Geometry check sheet. Reference: the model listing, model coordinates, mm. A direction names the side the tool comes from. Give positions to 0.01 mm unless a question says otherwise; leave off trailing zeros. Loops run counter-clockwise (first coordinate to the right, second up) from the corner with the lowest first, then second, coordinate; pieces in that order, holes last. Notation, with made-up numbers: (81.25, 9) - (140.25, 9) arc R18 ccw to (140.25, 13) - close; hole circle Ø11 at (73.5, 6.5). An arc over 180 degrees is marked (long way). Use a Markdown table: item, result. Add a question column.
1. Cross-section at D-D on x = 6.5. Enter the section's corners in (y, z).
2. Cross-section at A-A on x = 0. Enter the section's corners in (y, z), and give its area (3 significant figures).
3. Depth check by flat-ended pin: P1, Ø3, axis at y = 11.5, z = 14.5, coming from the +X side; P2, Ø5, axis at y = 6.5, z = 12.5, coming from the +X side; P3, Ø4, axis at x = -4.5, z = 3.5, coming from the +Y side. Enter the tip coordinate at first touch or a pass-through.
4. Cross-section at B-B on z = 6.75. Enter the section's corners in (x, y), and give its area (3 significant figures).
5. Draft check along Z on faces 5 (the flat face through (12, -9, 15.4)), 6 (the flat face through (-4, -4, 0)), 7 (the flat face through (13.16, -6.78, 19.34)). Enter one of: pulls with the +Z half, pulls with the -Z half, needs draft (parallel to the pull), parting line crosses it, or undercut.
6. Cross-section at C-C on y = -0.5. Enter the section's corners in (x, z).
7. Material ranges on L1, parallel to X at y = -0.5, z = 9.5; L2, parallel to Y at x = 0, z = 3.5; L3, parallel to Y at x = 0, z = 9.5, recorded low to high.
8. Set-up check for faces 1 (the flat face through (-15, 2.25, 19)), 2 (the cylindrical face through (13.94, -10.16, 19.34)), 3 (the flat face through (-15, -2.25, 19)), 4 (the flat face through (-12, -4, 5)): record each of +Z, -Z, +X, -X, +Y, -Y from which the full face is reachable in a straight line by a thin tool's end or side.
from build123d import *

# Parameters (mm, degrees)
F0_R     = 17.5
F0_R_2   = 5.5
F1_DEPTH = 5
F2_R     = 12.3
F2_R_2   = 5.5
F3_DEPTH = 10.4
F5_DEPTH = 8


with BuildPart() as f1:
    # F0 (on Top) → F1 (new body)
    with BuildSketch(Plane.XY):
        Circle(F0_R)
        Circle(F0_R_2, mode=Mode.SUBTRACT)
    extrude(amount=F1_DEPTH)

    # F2 (on face) → F3 (join)
    with BuildSketch(Plane.XY.offset(5)):
        Circle(F2_R)
        Circle(F2_R_2, mode=Mode.SUBTRACT)
    extrude(amount=F3_DEPTH)

    # F4 (on face) → F5 (join)
    with BuildSketch(Plane.XY.offset(15.4)):
        with BuildLine():
            Line((-1.5968973469, 12.1958976243), (-3.1451265822, 16.9608572537))
            ThreePointArc((-3.1451265822, 16.9608572537), (-5.330543153, 16.4057249061), (-7.4248809055, 15.5702807791))
            Line((-7.4248809055, 15.5702807791), (-5.8766516702, 10.8053211497))
            ThreePointArc((-5.8766516702, 10.8053211497), (-3.8009090308, 11.6979951504), (-1.5968973469, 12.1958976243))
        make_face()
        with BuildLine():
            ThreePointArc((-17.1026313765, 2.25), (-17.25, 0), (-17.1026313765, -2.25))
            Line((-17.1026313765, -2.25), (-12.0924563262, -2.25))
            ThreePointArc((-12.0924563262, -2.25), (-12.3, 0), (-12.0924563262, 2.25))
            Line((-12.0924563262, 2.25), (-17.1026313765, 2.25))
        make_face()
        with BuildLine():
            ThreePointArc((12.5138026145, -11.8729627358), (13.955543153, -10.139295602), (15.1588362498, -8.2323862612))
            Line((15.1588362498, -8.2323862612), (11.1055194893, -5.2874792552))
            ThreePointArc((11.1055194893, -5.2874792552), (9.9509090308, -7.2297586032), (8.4604858539, -8.9280557298))
            Line((8.4604858539, -8.9280557298), (12.5138026145, -11.8729627358))
        make_face()
        with BuildLine():
            Line((11.1055194893, -5.2874792552), (6.9247879586, -2.25))
            Line((6.9247879586, -2.25), (5.018714975, -2.25))
            ThreePointArc((5.018714975, -2.25), (4.4495934691, -3.2328188876), (3.6907453789, -4.077793343))
            Line((3.6907453789, -4.077793343), (4.2797543233, -5.8905764747))
            Line((4.2797543233, -5.8905764747), (8.4604858539, -8.9280557298))
            ThreePointArc((8.4604858539, -8.9280557298), (9.9509090308, -7.2297586032), (11.1055194893, -5.2874792552))
        make_face()
        with BuildLine():
            ThreePointArc((11.1055194893, -5.2874792552), (11.6979951504, -3.8009090308), (12.0924563262, -2.25))
            Line((12.0924563262, -2.25), (6.9247879586, -2.25))
            Line((6.9247879586, -2.25), (11.1055194893, -5.2874792552))
        make_face()
        with BuildLine():
            Line((6.9247879586, -2.25), (12.0924563262, -2.25))
            ThreePointArc((12.0924563262, -2.25), (12.2480041805, -1.1297759044), (12.3, 0))
            ThreePointArc((12.3, 0), (12.2480041805, 1.1297759044), (12.0924563262, 2.25))
            Line((12.0924563262, 2.25), (6.9247879586, 2.25))
            Line((6.9247879586, 2.25), (5.3827425223, 1.1296384104))
            ThreePointArc((5.3827425223, 1.1296384104), (5.4706070903, 0.5678539104), (5.5, 0))
            ThreePointArc((5.5, 0), (5.4706070903, -0.5678539104), (5.3827425223, -1.1296384104))
            Line((5.3827425223, -1.1296384104), (6.9247879586, -2.25))
        make_face()
        with BuildLine():
            Line((6.9247879586, 2.25), (12.0924563262, 2.25))
            ThreePointArc((12.0924563262, 2.25), (11.6979951504, 3.8009090308), (11.1055194893, 5.2874792552))
            Line((11.1055194893, 5.2874792552), (6.9247879586, 2.25))
        make_face()
        with BuildLine():
            Line((5.018714975, 2.25), (6.9247879586, 2.25))
            Line((6.9247879586, 2.25), (11.1055194893, 5.2874792552))
            ThreePointArc((11.1055194893, 5.2874792552), (9.9509090308, 7.2297586032), (8.4604858539, 8.9280557298))
            Line((8.4604858539, 8.9280557298), (4.2797543233, 5.8905764747))
            Line((4.2797543233, 5.8905764747), (3.6907453789, 4.077793343))
            ThreePointArc((3.6907453789, 4.077793343), (4.4495934691, 3.2328188876), (5.018714975, 2.25))
        make_face()
        with BuildLine():
            Line((4.2797543233, 5.8905764747), (8.4604858539, 8.9280557298))
            ThreePointArc((8.4604858539, 8.9280557298), (7.2297586032, 9.9509090308), (5.8766516702, 10.8053211497))
            Line((5.8766516702, 10.8053211497), (4.2797543233, 5.8905764747))
        make_face()
        with BuildLine():
            Line((2.737708887, 4.7702148851), (4.2797543233, 5.8905764747))
            Line((4.2797543233, 5.8905764747), (5.8766516702, 10.8053211497))
            ThreePointArc((5.8766516702, 10.8053211497), (3.8009090308, 11.6979951504), (1.5968973469, 12.1958976243))
            Line((1.5968973469, 12.1958976243), (0, 7.2811529494))
            Line((0, 7.2811529494), (0.5890089445, 5.4683698177))
            ThreePointArc((0.5890089445, 5.4683698177), (1.6995934691, 5.2308108396), (2.737708887, 4.7702148851))
        make_face()
        with BuildLine():
            Line((0, 7.2811529494), (1.5968973469, 12.1958976243))
            ThreePointArc((1.5968973469, 12.1958976243), (0, 12.3), (-1.5968973469, 12.1958976243))
            Line((-1.5968973469, 12.1958976243), (0, 7.2811529494))
        make_face()
        with BuildLine():
            Line((-0.5890089445, 5.4683698177), (0, 7.2811529494))
            Line((0, 7.2811529494), (-1.5968973469, 12.1958976243))
            ThreePointArc((-1.5968973469, 12.1958976243), (-3.8009090308, 11.6979951504), (-5.8766516702, 10.8053211497))
            Line((-5.8766516702, 10.8053211497), (-4.2797543233, 5.8905764747))
            Line((-4.2797543233, 5.8905764747), (-2.737708887, 4.7702148851))
            ThreePointArc((-2.737708887, 4.7702148851), (-1.6995934691, 5.2308108396), (-0.5890089445, 5.4683698177))
        make_face()
        with BuildLine():
            Line((-4.2797543233, 5.8905764747), (-5.8766516702, 10.8053211497))
            ThreePointArc((-5.8766516702, 10.8053211497), (-7.2297586032, 9.9509090308), (-8.4604858539, 8.9280557298))
            Line((-8.4604858539, 8.9280557298), (-4.2797543233, 5.8905764747))
        make_face()
        with BuildLine():
            Line((-3.6907453789, 4.077793343), (-4.2797543233, 5.8905764747))
            Line((-4.2797543233, 5.8905764747), (-8.4604858539, 8.9280557298))
            ThreePointArc((-8.4604858539, 8.9280557298), (-9.9509090308, 7.2297586032), (-11.1055194893, 5.2874792552))
            Line((-11.1055194893, 5.2874792552), (-6.9247879586, 2.25))
            Line((-6.9247879586, 2.25), (-5.018714975, 2.25))
            ThreePointArc((-5.018714975, 2.25), (-4.4495934691, 3.2328188876), (-3.6907453789, 4.077793343))
        make_face()
        with BuildLine():
            Line((-6.9247879586, 2.25), (-11.1055194893, 5.2874792552))
            ThreePointArc((-11.1055194893, 5.2874792552), (-11.6979951504, 3.8009090308), (-12.0924563262, 2.25))
            Line((-12.0924563262, 2.25), (-6.9247879586, 2.25))
        make_face()
        with BuildLine():
            Line((-12.0924563262, -2.25), (-6.9247879586, -2.25))
            Line((-6.9247879586, -2.25), (-5.3827425223, -1.1296384104))
            ThreePointArc((-5.3827425223, -1.1296384104), (-5.5, 0), (-5.3827425223, 1.1296384104))
            Line((-5.3827425223, 1.1296384104), (-6.9247879586, 2.25))
            Line((-6.9247879586, 2.25), (-12.0924563262, 2.25))
            ThreePointArc((-12.0924563262, 2.25), (-12.3, 0), (-12.0924563262, -2.25))
        make_face()
        with BuildLine():
            ThreePointArc((-12.0924563262, -2.25), (-11.6979951504, -3.8009090308), (-11.1055194893, -5.2874792552))
            Line((-11.1055194893, -5.2874792552), (-6.9247879586, -2.25))
            Line((-6.9247879586, -2.25), (-12.0924563262, -2.25))
        make_face()
        with BuildLine():
            Line((-8.4604858539, -8.9280557298), (-4.2797543233, -5.8905764747))
            Line((-4.2797543233, -5.8905764747), (-3.6907453789, -4.077793343))
            ThreePointArc((-3.6907453789, -4.077793343), (-4.4495934691, -3.2328188876), (-5.018714975, -2.25))
            Line((-5.018714975, -2.25), (-6.9247879586, -2.25))
            Line((-6.9247879586, -2.25), (-11.1055194893, -5.2874792552))
            ThreePointArc((-11.1055194893, -5.2874792552), (-9.9509090308, -7.2297586032), (-8.4604858539, -8.9280557298))
        make_face()
        with BuildLine():
            ThreePointArc((-8.4604858539, -8.9280557298), (-7.2297586032, -9.9509090308), (-5.8766516702, -10.8053211497))
            Line((-5.8766516702, -10.8053211497), (-4.2797543233, -5.8905764747))
            Line((-4.2797543233, -5.8905764747), (-8.4604858539, -8.9280557298))
        make_face()
        with BuildLine():
            Line((-1.5968973469, -12.1958976243), (0, -7.2811529494))
            Line((0, -7.2811529494), (-0.5890089445, -5.4683698177))
            ThreePointArc((-0.5890089445, -5.4683698177), (-1.6995934691, -5.2308108396), (-2.737708887, -4.7702148851))
            Line((-2.737708887, -4.7702148851), (-4.2797543233, -5.8905764747))
            Line((-4.2797543233, -5.8905764747), (-5.8766516702, -10.8053211497))
            ThreePointArc((-5.8766516702, -10.8053211497), (-3.8009090308, -11.6979951504), (-1.5968973469, -12.1958976243))
        make_face()
        with BuildLine():
            ThreePointArc((-1.5968973469, -12.1958976243), (0, -12.3), (1.5968973469, -12.1958976243))
            Line((1.5968973469, -12.1958976243), (0, -7.2811529494))
            Line((0, -7.2811529494), (-1.5968973469, -12.1958976243))
        make_face()
        with BuildLine():
            Line((5.8766516702, -10.8053211497), (4.2797543233, -5.8905764747))
            Line((4.2797543233, -5.8905764747), (2.737708887, -4.7702148851))
            ThreePointArc((2.737708887, -4.7702148851), (1.6995934691, -5.2308108396), (0.5890089445, -5.4683698177))
            Line((0.5890089445, -5.4683698177), (0, -7.2811529494))
            Line((0, -7.2811529494), (1.5968973469, -12.1958976243))
            ThreePointArc((1.5968973469, -12.1958976243), (3.8009090308, -11.6979951504), (5.8766516702, -10.8053211497))
        make_face()
        with BuildLine():
            ThreePointArc((5.8766516702, -10.8053211497), (7.2297586032, -9.9509090308), (8.4604858539, -8.9280557298))
            Line((8.4604858539, -8.9280557298), (4.2797543233, -5.8905764747))
            Line((4.2797543233, -5.8905764747), (5.8766516702, -10.8053211497))
        make_face()
        with BuildLine():
            Line((4.2797543233, -5.8905764747), (3.6907453789, -4.077793343))
            ThreePointArc((3.6907453789, -4.077793343), (3.2328188876, -4.4495934691), (2.737708887, -4.7702148851))
            Line((2.737708887, -4.7702148851), (4.2797543233, -5.8905764747))
        make_face()
        with BuildLine():
            Line((5.018714975, -2.25), (6.9247879586, -2.25))
            Line((6.9247879586, -2.25), (5.3827425223, -1.1296384104))
            ThreePointArc((5.3827425223, -1.1296384104), (5.2308108396, -1.6995934691), (5.018714975, -2.25))
        make_face()
        with BuildLine():
            Line((5.3827425223, 1.1296384104), (6.9247879586, 2.25))
            Line((6.9247879586, 2.25), (5.018714975, 2.25))
            ThreePointArc((5.018714975, 2.25), (5.2308108396, 1.6995934691), (5.3827425223, 1.1296384104))
        make_face()
        with BuildLine():
            ThreePointArc((2.737708887, 4.7702148851), (3.2328188876, 4.4495934691), (3.6907453789, 4.077793343))
            Line((3.6907453789, 4.077793343), (4.2797543233, 5.8905764747))
            Line((4.2797543233, 5.8905764747), (2.737708887, 4.7702148851))
        make_face()
        with BuildLine():
            ThreePointArc((-0.5890089445, 5.4683698177), (0, 5.5), (0.5890089445, 5.4683698177))
            Line((0.5890089445, 5.4683698177), (0, 7.2811529494))
            Line((0, 7.2811529494), (-0.5890089445, 5.4683698177))
        make_face()
        with BuildLine():
            ThreePointArc((-3.6907453789, 4.077793343), (-3.2328188876, 4.4495934691), (-2.737708887, 4.7702148851))
            Line((-2.737708887, 4.7702148851), (-4.2797543233, 5.8905764747))
            Line((-4.2797543233, 5.8905764747), (-3.6907453789, 4.077793343))
        make_face()
        with BuildLine():
            Line((-6.9247879586, 2.25), (-5.3827425223, 1.1296384104))
            ThreePointArc((-5.3827425223, 1.1296384104), (-5.2308108396, 1.6995934691), (-5.018714975, 2.25))
            Line((-5.018714975, 2.25), (-6.9247879586, 2.25))
        make_face()
        with BuildLine():
            Line((-6.9247879586, -2.25), (-5.018714975, -2.25))
            ThreePointArc((-5.018714975, -2.25), (-5.2308108396, -1.6995934691), (-5.3827425223, -1.1296384104))
            Line((-5.3827425223, -1.1296384104), (-6.9247879586, -2.25))
        make_face()
        with BuildLine():
            Line((-4.2797543233, -5.8905764747), (-2.737708887, -4.7702148851))
            ThreePointArc((-2.737708887, -4.7702148851), (-3.2328188876, -4.4495934691), (-3.6907453789, -4.077793343))
            Line((-3.6907453789, -4.077793343), (-4.2797543233, -5.8905764747))
        make_face()
        with BuildLine():
            Line((0, -7.2811529494), (0.5890089445, -5.4683698177))
            ThreePointArc((0.5890089445, -5.4683698177), (0, -5.5), (-0.5890089445, -5.4683698177))
            Line((-0.5890089445, -5.4683698177), (0, -7.2811529494))
        make_face()
    extrude(amount=F5_DEPTH)


solid = f1.part
Values found:
| question | item | result |
|---|---|---|
| 1 | outline | (-16.25, 0) - (16.25, 0) - (16.25, 5) - (10.44, 5) - (10.44, 23.4) - (-10.44, 23.4) - (-10.44, 5) - (-16.25, 5) - close |
| 2 | outline | (-17.5, 0) - (-5.5, 0) - (-5.5, 23.4) - (-12.3, 23.4) - (-12.3, 5) - (-17.5, 5) - close; (5.5, 0) - (17.5, 0) - (17.5, 5) - (12.3, 5) - (12.3, 23.4) - (5.5, 23.4) - close |
| 2 | area | 370 mm2 |
| 3 | P1 | stops at x = 7.16 |
| 3 | P2 | stops at x = 11.63 |
| 3 | P3 | stops at y = 17.32 |
| 4 | outline | circle Ø24.6 at (0, 0); hole circle Ø11 at (0, 0) |
| 4 | area | 380 mm2 |
| 5 | face 5 | undercut |
| 5 | face 6 | pulls with the -Z half |
| 5 | face 7 | needs draft |
| 6 | outline | (-17.49, 0) - (-5.48, 0) - (-5.48, 23.4) - (-17.24, 23.4) - (-17.24, 15.4) - (-12.29, 15.4) - (-12.29, 5) - (-17.49, 5) - close; (5.48, 0) - (17.49, 0) - (17.49, 5) - (12.29, 5) - (12.29, 23.4) - (5.48, 23.4) - close |
| 7 | L1 | x = -12.29 to -5.48, 5.48 to 12.29 |
| 7 | L2 | y = -17.5 to -5.5, 5.5 to 17.5 |
| 7 | L3 | y = -12.3 to -5.5, 5.5 to 12.3 |
| 8 | face 1 | +Z, -X, +Y |
| 8 | face 2 | +Z, +X, -Y |
| 8 | face 3 | +Z, -X, -Y |
| 8 | face 4 | none |
